from build123d import *

# Parameters (mm, degrees)
SKETCH1_W           = 406.4
SKETCH1_H           = 114.3
BOSS_EXTRUDE1_DEPTH = 12.7
CUT_EXTRUDE1_REACH  = 14.7
SKETCH2_R           = 10.4775


with BuildPart() as part:
    # Sketch1 → Boss-Extrude1 (new body)
    with BuildSketch(Plane(origin=(0, 0, 0), x_dir=(1, 0, 0), z_dir=(0, 1, 0))):
        with Locations((203.2, 57.15)):
            Rectangle(SKETCH1_W, SKETCH1_H)
    extrude(amount=BOSS_EXTRUDE1_DEPTH)

    # Sketch2 → Cut-Extrude1 (cut, up to next)
    with BuildSketch(Plane(origin=(0, 12.7, 0), x_dir=(1, 0, 0), z_dir=(0, 1, 0)), mode=Mode.PRIVATE) as cut_extrude1_sk1:
        with Locations((31.75, 31.75)):
            Circle(SKETCH2_R)
    cut_extrude1_tool1 = extrude(cut_extrude1_sk1.sketch, amount=-CUT_EXTRUDE1_REACH, mode=Mode.PRIVATE) & part.part
    add(cut_extrude1_tool1.solids().sort_by_distance((31.75, 12.7, -31.75))[0], mode=Mode.SUBTRACT)
    # Sketch2 → Cut-Extrude1 (cut, up to next)
    with BuildSketch(Plane(origin=(0, 12.7, 0), x_dir=(1, 0, 0), z_dir=(0, 1, 0)), mode=Mode.PRIVATE) as cut_extrude1_sk2:
        with Locations((374.65, 31.75)):
            Circle(SKETCH2_R)
    cut_extrude1_tool2 = extrude(cut_extrude1_sk2.sketch, amount=-CUT_EXTRUDE1_REACH, mode=Mode.PRIVATE) & part.part
    add(cut_extrude1_tool2.solids().sort_by_distance((374.65, 12.7, -31.75))[0], mode=Mode.SUBTRACT)


solid = part.part
Input: part model. Units: mm. Frame: model coordinates. Coordinates: 2 decimals unless noted, no trailing zeros. Loops run counter-clockwise (first coordinate to the right, second up) from the corner with the lowest first, then second, coordinate; pieces in that order, holes last. Notation, with made-up numbers: (32, 45) -> (47, 45) arc R3 ccw to (47, 49) -> close; hole circle Ø9 at (19.25, -27.75). An arc over 180 degrees is marked (long way). One line per item, written item: value.
(1) Draft query along X for faces 1 (the face through (200, 6, -114.3)), 2 (the face through (23.44, 6.44, -25.37)), 3 (the face through (0, 6, -56)). Return one class per face: pulls with the +X half, pulls with the -X half, needs draft (parallel to the pull), parting line crosses it, or undercut.
Answer below:
face 1: needs draft
face 2: undercut
face 3: pulls with the -X half
(2) Cut plane A-A (z = -31.75). Output: boundary loops of the cut face in (x, y).
Answer below:
outline: (0, 0) -> (21.27, 0) -> (21.27, 12.7) -> (0, 12.7) -> close; (42.23, 0) -> (364.17, 0) -> (364.17, 12.7) -> (42.23, 12.7) -> close; (385.13, 0) -> (406.4, 0) -> (406.4, 12.7) -> (385.13, 12.7) -> close
(3) Ray query, line 1 along X through (y, z) = (7.75, -31.75); line 2 along Z through (x, y) = (31.75, 6.5); line 3 along X through (y, z) = (5.5, -41). Return the intervals inside material, ascending.
Answer below:
line 1: x = 0 to 21.27, 42.23 to 364.17, 385.13 to 406.4
line 2: z = -114.3 to -42.23, -21.27 to 0
line 3: x = 0 to 26.83, 36.67 to 369.73, 379.57 to 406.4
(4) Cut plane B-B (x = 31.75). Output: boundary loops of the cut face in (y, z).
Answer below:
outline: (0, -114.3) -> (12.7, -114.3) -> (12.7, -42.23) -> (0, -42.23) -> close; (0, -21.27) -> (12.7, -21.27) -> (12.7, 0) -> (0, 0) -> close
